Geometry check sheet. Reference: the model listing, model coordinates, mm. A direction names the side the tool comes from. Give positions to 0.01 mm unless a question says otherwise; leave off trailing zeros. Order: outer loops, then holes, each group sorted by start corner. A loop starts at its lowest first (then second) coordinate and runs counter-clockwise, first axis right, second up. Notation, with made-up numbers: M 28.25,-1 L 38.25,-1 A18 cw 38.25,9 Z; hole C 16,1 d7. An arc over 180 degrees is marked long. Put each result on its own line as item: value. Start each with the question number.
Q1. Go/stop test with flat-tipped pins: pin 1 (1.5 mm diameter, centred on y = 1, z = 21, fed in from +X); pin 2 (1 mm diameter, centred on y = 8.5, z = 5.5, fed in from +X); pin 3 (1.5 mm diameter, centred on x = 2, z = 8, fed in from +Y). Record where each tip stops, or that it passes through.
Q2. Section check B-B on y = 0. Record the cut outline in (x, z), then the cut area to 3 significant figures.
Q3. Section check A-A on x = 0. Record the cut outline in (y, z).
Q4. Section check D-D on z = 1.5. Record the cut outline in (x, y).
Q5. Material ranges on L1, parallel to Z at x = 0, y = -18; L2, parallel to Z at x = -11.5, y = -3.5; L3, parallel to Y at x = 1.5, z = 10.5, recorded low to high.
Q6. Section check C-C on z = 10. Record the cut outline in (x, y), then the cut area to 3 significant figures.
Q7. Mould release check, pull along X, two halves, no side actions. Record for faces 1 (the flat face through (13.1, -4.2, 25)), 2 (the cylindrical face through (-4.336, -19.524, 12.832)), 3 (the cylindrical face through (-3.996, -15.891, 16.676)), 4 (the cylindrical face through (6.75, 10.58, 14.63)): +X half, -X half, draft (parallel to the pull), parting line (faces both ways), or undercut.
Q8. Access from +Z, -Z, +X, -X, +Y, -Y to the whole of each face (thin tool, end or side, straight path). Record for faces 5 (the flat face through (0, 0, 0)), 6 (the flat face through (0, 0, 5)).
```python
from build123d import *

# Parameters (mm, degrees)
F0_R     = 20
F1_DEPTH = 25
F2_R     = 12.55
F3_DEPTH = 20
F4_R     = 4
F5_DEPTH = 25
F6_SIZE  = 1


with BuildPart() as f1:
    # F0 (on Top) → F1 (new body)
    with BuildSketch(Plane.XY):
        Circle(F0_R)
    extrude(amount=F1_DEPTH)

    # F2 (on face) → F3 (cut)
    with BuildSketch(Plane.XY.offset(25)):
        Circle(F2_R)
    extrude(amount=-F3_DEPTH, mode=Mode.SUBTRACT)

    # F4 (on Front) → F5 (cut)
    with BuildSketch(Plane.XZ):
        with Locations((0, 16.5)):
            Circle(F4_R)
    extrude(amount=F5_DEPTH, mode=Mode.SUBTRACT)

    # F6
    f6_edges = [f1.edges().sort_by_distance(p)[0] for p in [
        (-20, 0, 0),
        (-12.55, 0, 25),
    ]]
    chamfer(f6_edges, length=F6_SIZE)


solid = f1.part
```
Results found:
1. pin 1: stops at x = 20
1. pin 2: stops at x = 18.33
1. pin 3: stops at y = 19.96
2. outline: M -20,1 L -19,0 L 19,0 L 20,1 L 20,25 L 13.55,25 L 12.55,24 L 12.55,5 L -12.55,5 L -12.55,24 L -13.55,25 L -20,25 Z
2. area: 496 mm^2
3. outline: M -20,1 L -19,0 L 19,0 L 20,1 L 20,25 L 13.55,25 L 12.55,24 L 12.55,5 L -12.55,5 L -12.55,12.5 L -20,12.5 Z; M -20,20.5 L -12.55,20.5 L -12.55,24 L -13.55,25 L -20,25 Z
4. outline: C 0,0 d40
5. L1: z = 0 to 12.5, 20.5 to 25
5. L2: z = 0 to 5
5. L3: y = -19.94 to -12.46, 12.46 to 19.94
6. outline: C 0,0 d40; hole C 0,0 d25.1
6. area: 762 mm^2
7. face 1: draft
7. face 2: parting line
7. face 3: undercut
7. face 4: undercut
8. face 5: -Z, +X, -X, +Y, -Y
8. face 6: +Z
